from build123d import *

# Parameters (mm, degrees)
BOSS_EXTRUDE1_DEPTH = 31
SKETCH4_W           = 25
SKETCH4_H           = 15
CUT_EXTRUDE2_DEPTH  = 25
CUT_EXTRUDE4_DEPTH  = 11.5
SKETCH7_W           = 31
SKETCH7_H           = 1.7
BOSS_EXTRUDE3_DEPTH = 7
BOSS_EXTRUDE4_DEPTH = 7
LPATTERN1_COUNT     = 8
LPATTERN1_PITCH     = 4
SKETCH11_W          = 12
SKETCH11_H          = 6.5
BOSS_EXTRUDE5_DEPTH = 5.5
FILLET5_R           = 3
SKETCH12_W          = 12
SKETCH12_H          = 6.5
BOSS_EXTRUDE6_DEPTH = 6
CUT_EXTRUDE5_DEPTH  = 12
FILLET6_R           = 2


with BuildPart() as part:
    # Sketch1 → Boss-Extrude1 (new body)
    with BuildSketch(Plane.XY):
        Polygon((0, 0), (0, -30), (12, -30), (12, -20), (5, 0), align=None)
    extrude(amount=-BOSS_EXTRUDE1_DEPTH)

    # Sketch4 → Cut-Extrude2 (cut)
    with BuildSketch(Plane.ZY):
        with Locations((-15, -24.143402944)):
            Rectangle(SKETCH4_W, SKETCH4_H)
    extrude(amount=-CUT_EXTRUDE2_DEPTH, mode=Mode.SUBTRACT)

    # Sketch6 → Cut-Extrude4 (cut, symmetric)
    with BuildSketch(Plane.XY.offset(-15.25)):
        Polygon((5, 0), (5, -14), (9.9, -14), align=None)
    extrude(amount=CUT_EXTRUDE4_DEPTH, both=True, mode=Mode.SUBTRACT)

    # Sketch7 → Boss-Extrude3 (add)
    with BuildSketch(Plane(origin=(0, -25.5, 0), x_dir=(1, 0, 0), z_dir=(0, 1, 0))):
        with Locations((-4.2231607, 26.8)):
            Rectangle(SKETCH7_W, SKETCH7_H)
    extrude(amount=BOSS_EXTRUDE3_DEPTH)

    # Sketch10 → Boss-Extrude4 (add)
    with BuildSketch(Plane(origin=(0, -25.5, 0), x_dir=(1, 0, 0), z_dir=(0, 1, 0))):
        with BuildLine():
            Line((10.229764516, 21.588776044), (9.674536509, 21.588776044))
            ThreePointArc((9.674536509, 21.588776044), (9.015771799, 23.054925169), (9.300491414, 24.636854036))
            ThreePointArc((9.300491414, 24.636854036), (8.903062553, 25.310703075), (8.452150513, 25.95))
            Line((8.452150513, 25.95), (11.452150513, 25.95))
            ThreePointArc((11.452150513, 25.95), (11.001238473, 25.310703075), (10.603809612, 24.636854036))
            ThreePointArc((10.603809612, 24.636854036), (10.888529227, 23.054925169), (10.229764516, 21.588776044))
        make_face()
    boss_extrude4 = extrude(amount=BOSS_EXTRUDE4_DEPTH)

    # LPattern1: Boss-Extrude4 ×8
    with Locations(*[(-i * LPATTERN1_PITCH, 0, 0) for i in range(1, LPATTERN1_COUNT)]):
        add(boss_extrude4)

    # Sketch11 → Boss-Extrude5 (add)
    with BuildSketch(Plane(origin=(0, 0, -31), x_dir=(-1, 0, 0), z_dir=(0, 0, -1))):
        with Locations((-6, -26.75)):
            Rectangle(SKETCH11_W, SKETCH11_H)
    extrude(amount=BOSS_EXTRUDE5_DEPTH)

    # Fillet5
    # the kernel refuses this fillet: 3 mm, written as the material it adds along each edge
    with BuildSketch(Plane(origin=(5, -14, -34.25), x_dir=(0, 1, 0), z_dir=(0, 0, 1))) as fillet5_piece_1_section:
        with BuildLine():
            CenterArc((FILLET5_R, -FILLET5_R), FILLET5_R, 90, 90)
            Line((0, -FILLET5_R), (0, 0))
            Line((0, 0), (FILLET5_R, 0))
        make_face()
    fillet5_piece_1 = extrude(amount=38, mode=Mode.PRIVATE)
    fillet5_piece_1 = split(fillet5_piece_1, bisect_by=Plane(origin=(5.670103817, -13.329896183, -31), z_dir=(0, 0, 1)), keep=Keep.TOP, mode=Mode.PRIVATE)
    fillet5_piece_1 = split(fillet5_piece_1, bisect_by=Plane(origin=(5.670103817, -13.329896183, 0), z_dir=(0, 0, -1)), keep=Keep.TOP, mode=Mode.PRIVATE)
    add(fillet5_piece_1)
    with BuildSketch(Plane(origin=(0, -16.643402944, -2.5), x_dir=(0, -1, 0), z_dir=(1, 0, 0))) as fillet5_piece_2_section:
        with BuildLine():
            CenterArc((FILLET5_R, FILLET5_R), FILLET5_R, 180, 90)
            Line((0, FILLET5_R), (0, 0))
            Line((0, 0), (FILLET5_R, 0))
        make_face()
    fillet5_piece_2 = extrude(amount=18.32519103, mode=Mode.PRIVATE)
    fillet5_piece_2 = split(fillet5_piece_2, bisect_by=Plane(origin=(10.459559167, -15.598740478, -3.164212855), z_dir=(-0.9438583563660173, -0.33035042472810633, 0)), keep=Keep.TOP, mode=Mode.PRIVATE)
    add(fillet5_piece_2)
    with BuildSketch(Plane(origin=(0, -16.643402944, -27.5), x_dir=(0, 0, 1), z_dir=(1, 0, 0))) as fillet5_piece_3_section:
        with BuildLine():
            CenterArc((FILLET5_R, FILLET5_R), FILLET5_R, 180, 90)
            Line((0, FILLET5_R), (0, 0))
            Line((0, 0), (FILLET5_R, 0))
        make_face()
    fillet5_piece_3 = extrude(amount=18.32519103, mode=Mode.PRIVATE)
    fillet5_piece_3 = split(fillet5_piece_3, bisect_by=Plane(origin=(10.435387917, -15.529679764, -26.806522223), z_dir=(-0.9438583563660173, -0.33035042472810633, 0)), keep=Keep.TOP, mode=Mode.PRIVATE)
    add(fillet5_piece_3)

    # Sketch12 → Boss-Extrude6 (add)
    with BuildSketch(Plane.XY):
        with Locations((6, -26.75)):
            Rectangle(SKETCH12_W, SKETCH12_H)
    extrude(amount=BOSS_EXTRUDE6_DEPTH)

    # Sketch13 → Cut-Extrude5 (cut)
    with BuildSketch(Plane.ZY):
        Polygon((-34.3, -25.5), (-27.5, -25.5), (-27.5, -32.069121633), (-31.5, -32.069121633), (-31.5, -29), (-34.3, -29), align=None)
        Polygon((1.387837299, -29), (4.187837299, -29), (4.187837299, -25.5), (-2.612162701, -25.5), (-2.612162701, -32.069121633), (1.387837299, -32.069121633), align=None)
    extrude(amount=-CUT_EXTRUDE5_DEPTH, mode=Mode.SUBTRACT)

    # Fillet6
    fillet6_edges = [part.edges().sort_by_distance(p)[0] for p in [
        (6, -23.5, -31),
        (6, -23.5, -36.5),
        (6, -23.5, 0),
        (6, -23.5, 6),
    ]]
    fillet(fillet6_edges, radius=FILLET6_R)


solid = part.part
Check sheet for the modelled part. Datum: model origin and axes. Units: mm. A direction names the side the tool comes from. Give positions to 0.01 mm unless a question says otherwise; leave off trailing zeros. Loops run counter-clockwise (first coordinate to the right, second up) from the corner with the lowest first, then second, coordinate; pieces in that order, holes last. Notation, with made-up numbers: M 63,52.5 L 73,52.5 A14 cw 73,57.5 Z; hole C 65.5,25 d11. An arc over 180 degrees is marked long. Use a Markdown table: item, result. Add a question column.
Q1. Sectioned sample at B-B, the plane z = -6.5. Record the cut outline in (x, y), then the cut area to 3 significant figures.
Q2. Mould release check, pull along X, two halves, no side actions. Record for faces 1 (the cylindrical face through (5.92, -24.1, -35.93)), 2 (the cylindrical face through (10.89, -22.05, -23.08)), 3 (the flat face through (-4, -22, -25.95)): pulls with the +X half, pulls with the -X half, needs draft (parallel to the pull), parting line crosses it, or undercut.
Q3. Scan lines: line 1 along Z through (x, y) = (6, -4.5); line 2 along Z through (x, y) = (4, -20.75); line 3 along Y through (x, z) = (2.5, -21.5). Record each from-to range of solid material in increasing order. Write a range as [from, to].
Q4. Go/stop test with flat-tipped pins: pin 1 (6 mm diameter, centred on y = -5.5, z = -7, fed in from +X); pin 2 (4 mm diameter, centred on y = -12.5, z = -2, fed in from -X); pin 3 (2 mm diameter, centred on x = -14.5, y = -23.5, fed in from -Z). Record where each tip stops, or that it passes through.
Q5. Sectioned sample at D-D, the plane z = -30. Record the cut outline in (x, y), then the cut area to 3 significant figures.
Q6. Sectioned sample at A-A, the plane y = -27. Record the cut outline in (x, z), then the cut area to 3 significant figures.
Q7. Sectioned sample at C-C, the plane y = -9. Record the cut outline in (x, z), then the cut area to 3 significant figures.
Q8. Tool access check on faces 4 (the flat face through (6, -25.5, 1)), 5 (the flat face through (-8, -22, -25.95)), 6 (the flat face through (-10, -22, -27.65)), 7 (the cylindrical face through (3.007, -22.049, -25.32)), 8 (the cylindrical face through (-2.98, -22.05, -23.03)). Record the directions out of +Z, -Z, +X, -X, +Y, -Y that give a thin tool (end or side, any length) a straight path to the whole face; none if there is none.
Verdict:
| question | item | result |
|---|---|---|
| 1 | outline | M 0,-16.64 L 10.83,-16.64 L 9.9,-14 L 8,-14 A3 cw 5,-11 L 5,0 L 0,0 Z |
| 1 | area | 99.3 mm^2 |
| 2 | face 1 | needs draft |
| 2 | face 2 | pulls with the +X half |
| 2 | face 3 | undercut |
| 3 | line 1 | [-31, -26.75], [-3.75, 0] |
| 3 | line 2 | [-31, -25.95], [-2.5, 0] |
| 3 | line 3 | [-16.64, 0] |
| 4 | pin 1 | x = 5 |
| 4 | pin 2 | x = 0 |
| 4 | pin 3 | z = -27.65 |
| 5 | outline | M 0,-25.5 L 12,-25.5 L 12,-20 L 5,0 L 0,0 Z |
| 5 | area | 236 mm^2 |
| 6 | outline | M 0,-36.5 L 12,-36.5 L 12,-34.3 L 0,-34.3 Z; M 0,4.19 L 12,4.19 L 12,6 L 0,6 Z |
| 6 | area | 48.1 mm^2 |
| 7 | outline | M 0,-31 L 8.15,-31 L 8.15,-26.75 L 5,-26.75 L 5,-3.75 L 8.15,-3.75 L 8.15,0 L 0,0 Z |
| 7 | area | 180 mm^2 |
| 8 | face 4 | +X, -X |
| 8 | face 5 | +Z, +Y, -Y |
| 8 | face 6 | -Z, -X, +Y, -Y |
| 8 | face 7 | -Y |
| 8 | face 8 | +Y, -Y |
